For this review, use the dimensioned drawing (mm, ordinates from the lowest corner) and the shaded views. Coordinates: 2 decimals unless noted, no trailing zeros. Order: outer loops, then holes, each group sorted by start corner. A loop starts at its lowest first (then second) coordinate and runs counter-clockwise, first axis right, second up. Notation, with made-up numbers: M -20.75,67 L 13.25,67 A10 ccw 13.25,79 Z; hole C -7.5,-23.5 d8. An arc over 180 degrees is marked long. Answer in a Markdown table with one row per item.
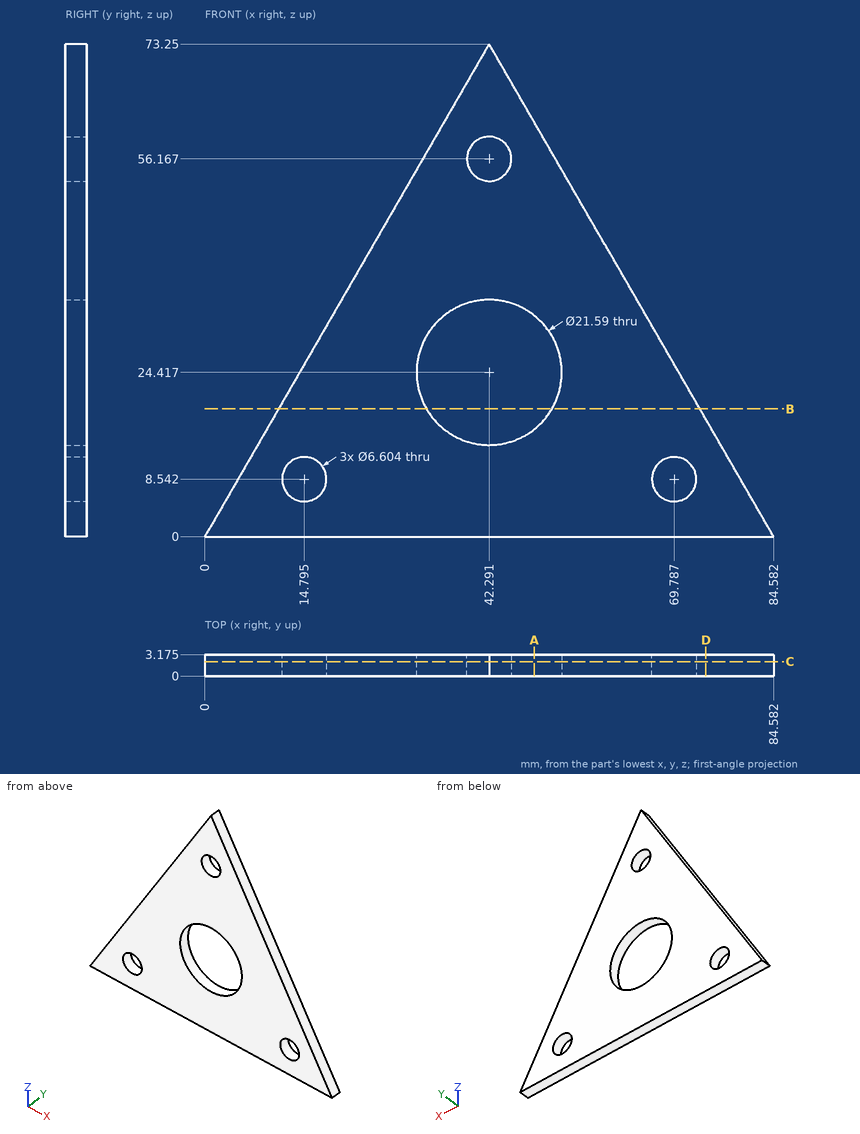
(1) Insertion check: pin 1 Ø1 at (x, y) = (32.5, 0.5) entering from +Z. The pin has a flat end and moves straight along its axis. Give the tip position at first contact, or say it passes through.
Return value:
| item | result |
|---|---|
| pin 1 | stops at z = 57.16 |
(2) For line 1 along Z through (x, y) = (43.5, 1.75) (1 decimal); line 2 along Z through (x, y) = (36.5, 1.6) (1 decimal); line 3 along X through (y, z) = (1.1, 32) (1 decimal), list the stretches that pass through material, from the lowest coordinate up. Write a range as from..to.
Return value:
| item | result |
|---|---|
| line 1 | z = 0..13.7, 35.1..53.1, 59.2..71.2 |
| line 2 | z = 0..15.3, 33.5..63.2 |
| line 3 | x = 18.5..34.6, 50..66.1 |
(3) Add section D-D, the plane x = 74.5. Give the boundary of the cut face in (y, z) (1 decimal).
Return value:
| item | result |
|---|---|
| outline | M 0,0 L 3.2,0 L 3.2,17.5 L 0,17.5 Z |
(4) Add section A-A, the plane x = 49. Give the boundary of the cut face in (y, z) (1 decimal).
Return value:
| item | result |
|---|---|
| outline | M 0,0 L 3.2,0 L 3.2,16 L 0,16 Z; M 0,32.9 L 3.2,32.9 L 3.2,61.6 L 0,61.6 Z |
(5) Add section C-C, the plane y = 2.15. Give the number of separate pieces and of enclosed holes in the cut face, and give its area (3 significant figures).
Return value:
| item | result |
|---|---|
| separate pieces | 1 |
| enclosed holes | 4 |
| area | 2,630 mm2 |
(6) Add section B-B, the plane z = 19. Give the boundary of the cut face in (x, y) (1 decimal).
Return value:
| item | result |
|---|---|
| outline | M 11,0 L 33,0 L 33,3.2 L 11,3.2 Z; M 51.6,0 L 73.6,0 L 73.6,3.2 L 51.6,3.2 Z |
